Input: part model. Units: mm. Frame: model coordinates. A direction names the side the tool comes from. Round coordinates to 2 decimals unless told otherwise and drop trailing zeros. Order: outer loops, then holes, each group sorted by start corner. A loop starts at its lowest first (then second) coordinate and runs counter-clockwise, first axis right, second up.
Item 1: Mould query, pull axis Y, two halves, no side actions, for faces 1 (the flat face through (7.736, -1, -49)), 2 (the flat face through (20.911, -1, -49)), 3 (the flat face through (16, -9.419, -49)). Classes: released by +Y, released by -Y, zero draft, split by the parting line, or undercut.
Item 2: Cut plane B-B on x = 17. Output: boundary loops of the cut face in (y, z), then the cut area to 3 significant figures.
Item 3: First-contact query: pin 1 (6 mm diameter, centred on x = 11, y = -0.5, fed in from +Z). Flat tip, straight axial feed; report the tip coordinate or a pass-through.
Item 4: Cut plane A-A on z = -54. Output: boundary loops of the cut face in (x, y).
Item 5: Reachability of faces 4 (the flat face through (16, -5.744, -49)), 5 (the flat face through (10, -1, -100)) from +Z, -Z, +X, -X, +Y, -Y: full face, straight path, thin tool, end or side. Return the list, or none.
Item 6: Cut plane C-C on y = -4.75. Output: boundary loops of the cut face in (x, z).
Item 7: Line query: L1, parallel to X at y = -2, z = -94; L2, parallel to Y at x = 18.25, z = -92.5. Output: solid intervals per line, ascending.
```python
from build123d import *

# Parameters (mm, degrees)
SKETCH1_W           = 16.85
SKETCH1_H           = 16.85
SKETCH1_W_2         = 9.5
SKETCH1_H_2         = 9.5
BOSS_EXTRUDE1_DEPTH = 100


with BuildPart() as part:
    # Sketch1 → Boss-Extrude1 (new body)
    with BuildSketch(Plane.XY):
        with Locations((16.160752053, -0.994216696)):
            Rectangle(SKETCH1_W, SKETCH1_H)
        with Locations((16.160752053, -0.994216696)):
            Rectangle(SKETCH1_W_2, SKETCH1_H_2, mode=Mode.SUBTRACT)
    extrude(amount=-BOSS_EXTRUDE1_DEPTH)


solid = part.part
```
From the geometry:
1. face 1: zero draft
1. face 2: undercut
1. face 3: released by -Y
2. outline: (-9.42, -100) - (-5.74, -100) - (-5.74, 0) - (-9.42, 0) - close; (3.76, -100) - (7.43, -100) - (7.43, 0) - (3.76, 0) - close
2. area: 735 mm2
3. pin 1: stops at z = 0
4. outline: (7.74, -9.42) - (24.59, -9.42) - (24.59, 7.43) - (7.74, 7.43) - close; hole (11.41, -5.74) - (20.91, -5.74) - (20.91, 3.76) - (11.41, 3.76) - close
5. face 4: +Z, -Z
5. face 5: -Z, +X, -X, +Y, -Y
6. outline: (7.74, -100) - (11.41, -100) - (11.41, 0) - (7.74, 0) - close; (20.91, -100) - (24.59, -100) - (24.59, 0) - (20.91, 0) - close
7. L1: x = 7.74 to 11.41, 20.91 to 24.59
7. L2: y = -9.42 to -5.74, 3.76 to 7.43
